Verification items for the finished model (mm, model axes). Face numbers are marked on the shaded views. A direction names the side the tool comes from. Round coordinates to 2 decimals unless told otherwise and drop trailing zeros. Write each loop counter-clockwise with the first axis right and the second up, starting at its lowest first coordinate (ties: lowest second). Pieces come first, ordered by that corner, then holes. Notation, with made-up numbers: M 41,23 L 85,23 A27 ccw 85,52 Z; hole C 38.5,8 d5. An arc over 180 degrees is marked long. One line per question, with ' | ' between items. Start each with the question number.
Q1. Cross-section at A-A (x = 0). Record the boundary of the cut face in (y, z), then the cut area to 3 significant figures.
Q2. Cross-section at D-D (x = 26). Record the boundary of the cut face in (y, z), then the cut area to 3 significant figures.
Q3. Thickness scan on line 1 along X through (y, z) = (47, 0); line 2 along Y through (x, z) = (14.5, 22); line 3 along Z through (x, y) = (2.5, 14.5). Record the ranges inside material, lowest first. Write a range as from..to.
Q4. Cross-section at B-B (z = 3). Record the boundary of the cut face in (x, y).
Q5. Tool access check on the marked faces 1 and 2. Record the directions out of +Z, -Z, +X, -X, +Y, -Y that give a thin tool (end or side, any length) a straight path to the whole face; none if there is none.
Q6. Cross-section at C-C (y = 3.8). Record the boundary of the cut face in (x, z), then the cut area to 3 significant figures.
Q7. Gauge pin test, flat ends, axial feed: pin 1 (1.5 mm diameter, centred on x = -18.5, z = -3.5, fed in from +Y); pin 2 (9 mm diameter, centred on x = -2.5, z = -38.5, fed in from +Y); pin 3 (1.5 mm diameter, centred on y = 10.5, z = 2.5, fed in from +X). Record the tip position at first contact, or that the pin passes through.
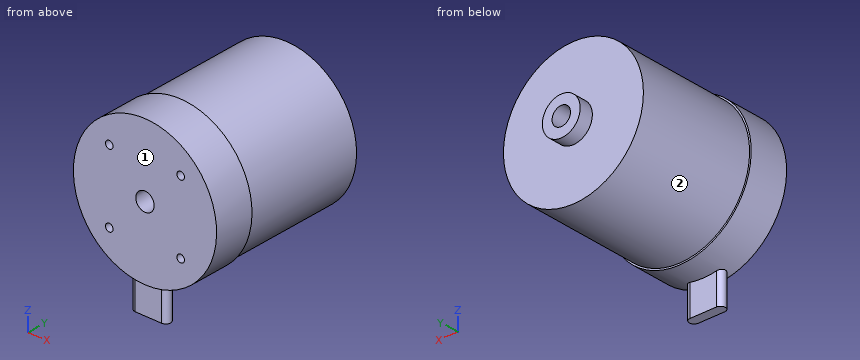
from build123d import *

# Parameters (mm, degrees)
SKETCH3_R           = 1.65
CUT_EXTRUDE1_DEPTH  = 5
BOSS_EXTRUDE1_START = -2
BOSS_EXTRUDE1_DEPTH = 15


with BuildPart() as part:
    # Sketch2 → Revolve1 (revolve)
    with BuildSketch(Plane.XY, mode=Mode.PRIVATE) as revolve1_sk:
        Polygon((4, 0), (4, 76), (8.25, 76), (8.25, 70), (30.5, 70), (30.5, 17.5), (31.2, 17.5), (31.2, 0), align=None)
    revolve(revolve1_sk.sketch.rotate(Axis((0, 0, 0), (0, 1, 0)), 90), axis=Axis((0, 0, 0), (0, 1, 0)))

    # Sketch3 → Cut-Extrude1 (cut)
    with BuildSketch(Plane.XZ):
        with Locations(Location((15.556349186, -15.556349186, 0), (0, 0, 270))):
            Circle(SKETCH3_R)
        with Locations(Location((-15.556349186, -15.556349186, 0), (0, 0, 270))):
            Circle(SKETCH3_R)
        with Locations(Location((-15.556349186, 15.556349186, 0), (0, 0, 270))):
            Circle(SKETCH3_R)
        with Locations(Location((15.556349186, 15.556349186, 0), (0, 0, 270))):
            Circle(SKETCH3_R)
    extrude(amount=-CUT_EXTRUDE1_DEPTH, mode=Mode.SUBTRACT)

    # Sketch4 → Boss-Extrude1 (add)
    with BuildSketch(Plane(origin=(0, 0, -31.2), x_dir=(-1, 0, 0), z_dir=(0, 0, -1)).offset(BOSS_EXTRUDE1_START)):
        with BuildLine():
            Line((-5.75, 5.9), (5.75, 5.9))
            ThreePointArc((5.75, 5.9), (7.85, 3.8), (5.75, 1.7))
            Line((5.75, 1.7), (-5.75, 1.7))
            ThreePointArc((-5.75, 1.7), (-7.85, 3.8), (-5.75, 5.9))
        make_face()
    extrude(amount=BOSS_EXTRUDE1_DEPTH)


solid = part.part
Determined:
1) outline: M 0,-31.2 L 1.7,-31.2 L 1.7,-44.2 L 5.9,-44.2 L 5.9,-31.2 L 17.5,-31.2 L 17.5,-30.5 L 70,-30.5 L 70,-8.25 L 76,-8.25 L 76,-4 L 0,-4 Z; M 0,4 L 76,4 L 76,8.25 L 70,8.25 L 70,30.5 L 17.5,30.5 L 17.5,31.2 L 0,31.2 Z | area: 3,840 mm²
2) outline: M 0,-17.25 L 17.5,-17.25 L 17.5,-15.95 L 70,-15.95 L 70,15.95 L 17.5,15.95 L 17.5,17.25 L 0,17.25 Z | area: 2,280 mm²
3) line 1: x = -30.5..-4, 4..30.5 | line 2: y = 0..70 | line 3: z = -31.1..-3.12, 3.12..31.1
4) outline: M -31.06,0 L -2.65,0 L -2.65,76 L -7.69,76 L -7.69,70 L -30.35,70 L -30.35,17.5 L -31.06,17.5 Z; M 2.65,0 L 31.06,0 L 31.06,17.5 L 30.35,17.5 L 30.35,70 L 7.69,70 L 7.69,76 L 2.65,76 Z
5) face 1: +Z, -Z, +X, -X, -Y | face 2: +Y
6) outline: M -7.85,-44.2 L 7.85,-44.2 L 7.85,-30.2 A31.2 ccw long -7.85,-30.2 Z; hole C -15.56,-15.56 d3.3; hole C -15.56,15.56 d3.3; hole C 0,0 d8; hole C 15.56,-15.56 d3.3; hole C 15.56,15.56 d3.3 | area: 3,180 mm²
7) pin 1: stops at y = 70 | pin 2: stops at y = 5.9 | pin 3: stops at x = 31.15
